Geometry: final body of the model. Coordinates: model frame, mm. A direction names the side the tool comes from. Give positions to 0.01 mm unless a question says otherwise; leave off trailing zeros.
1. First-contact query: P1, Ø4.5, axis at x = 0, y = 33.75, coming from the +Z side; P2, Ø3, axis at x = -22, z = 4, coming from the +Y side; P3, Ø2, axis at x = 6.5, z = 4, coming from the +Y side. Flat tips, straight axial feed; report the tip coordinate or a pass-through.
2. Material intervals for line 1 along Y through (x, z) = (-15.5, 9.25); line 2 along X through (y, z) = (-17, 5); line 3 along X through (y, z) = (-14.5, 2.5), sorted ascending.
3. Section A-A, the plane y = 0. State how many separate pieces and enclosed holes the cut face has, then the cut area to 3 significant figures.
4. Access query for faces 1 (the face through (14.7, -14, 3.3)), 2 (the face through (17.895, -17.697, 8.324)). Directions: +Z, -Z, +X, -X, +Y, -Y. A direction counts if a zero-diameter tool reaches every point of the face in a straight line with its end or side. Return the directions, or none.
5. Draft query along X for faces 3 (the face through (-1, -17, 10)), 4 (the face through (-14.7, 14, 3.3)). Return one class per face: +X half, -X half, draft (parallel to the pull), parting line (faces both ways), or undercut.
from build123d import *

# Parameters (mm, degrees)
SKIZZE3_R                       = 42.5
AUFSATZ_LINEAR_AUSTRAGEN1_DEPTH = 10
SKIZZE4_R                       = 10
SCHNITT_LINEAR_AUSTRAGEN1_DEPTH = 10
SKIZZE5_R                       = 3.25
SCHNITT_LINEAR_AUSTRAGEN3_DEPTH = 3.4
SKIZZE6_R                       = 1.7
SCHNITT_LINEAR_AUSTRAGEN4_DEPTH = 6.6
KREISMUSTER1_COUNT              = 4
SKIZZE7_R                       = 13.1
SCHNITT_LINEAR_AUSTRAGEN5_DEPTH = 9
VERRUNDUNG1_R                   = 4
FASE1_SIZE                      = 2


with BuildPart() as part:
    # Skizze3 → Aufsatz-Linear austragen1 (new body)
    with BuildSketch(Plane.XY):
        Circle(SKIZZE3_R)
    extrude(amount=AUFSATZ_LINEAR_AUSTRAGEN1_DEPTH)

    # Skizze4 → Schnitt-Linear austragen1 (cut)
    with BuildSketch(Plane.XY.offset(10)):
        Circle(SKIZZE4_R)
    extrude(amount=-SCHNITT_LINEAR_AUSTRAGEN1_DEPTH, mode=Mode.SUBTRACT)

    # Skizze5 → Schnitt-Linear austragen3 (cut)
    with BuildSketch(Plane.XY.offset(10)):
        with Locations((-15.5, 15.5)):
            Circle(SKIZZE5_R)
        with Locations((-33.75, 0)):
            Circle(SKIZZE5_R)
    schnitt_linear_austragen3 = extrude(amount=-SCHNITT_LINEAR_AUSTRAGEN3_DEPTH, mode=Mode.SUBTRACT)

    # Skizze6 → Schnitt-Linear austragen4 (cut)
    with BuildSketch(Plane.XY.offset(6.6)):
        with Locations((-15.5, 15.5)):
            Circle(SKIZZE6_R)
        with Locations((-33.75, 0)):
            Circle(SKIZZE6_R)
    schnitt_linear_austragen4 = extrude(amount=-SCHNITT_LINEAR_AUSTRAGEN4_DEPTH, mode=Mode.SUBTRACT)

    # Kreismuster1: Schnitt-Linear austragen3, Schnitt-Linear austragen4 ×4 about axis
    kreismuster1_axis = Axis((0, 0, 0), (0, 0, 1))
    add([schnitt_linear_austragen3.rotate(kreismuster1_axis, i * 360 / KREISMUSTER1_COUNT) for i in range(1, KREISMUSTER1_COUNT)], mode=Mode.SUBTRACT)
    add([schnitt_linear_austragen4.rotate(kreismuster1_axis, i * 360 / KREISMUSTER1_COUNT) for i in range(1, KREISMUSTER1_COUNT)], mode=Mode.SUBTRACT)

    # Skizze7 → Schnitt-Linear austragen5 (cut)
    with BuildSketch(Plane.XY.offset(10)):
        Circle(SKIZZE7_R)
    extrude(amount=-SCHNITT_LINEAR_AUSTRAGEN5_DEPTH, mode=Mode.SUBTRACT)

    # Verrundung1
    verrundung1_edges = [part.edges().sort_by_distance(p)[0] for p in [
        (-42.5, 0, 10),
    ]]
    fillet(verrundung1_edges, radius=VERRUNDUNG1_R)

    # Fase1
    fase1_edges = [part.edges().sort_by_distance(p)[0] for p in [
        (-13.1, 0, 10),
    ]]
    chamfer(fase1_edges, length=FASE1_SIZE)


solid = part.part
Answers below:
1. P1: stops at z = 6.6
1. P2: stops at y = 37.23
1. P3: stops at y = 42.14
2. line 1: y = -37.78 to -18.75, -12.25 to 12.25, 18.75 to 37.78
2. line 2: x = -38.95 to -16.3, -14.7 to 14.7, 16.3 to 38.95
2. line 3: x = -39.95 to -16.87, -14.13 to 14.13, 16.87 to 39.95
3. separate pieces: 4
3. enclosed holes: 0
3. area: 494 mm2
4. face 1: +Z, -Z
4. face 2: +Z
5. face 3: draft
5. face 4: undercut
